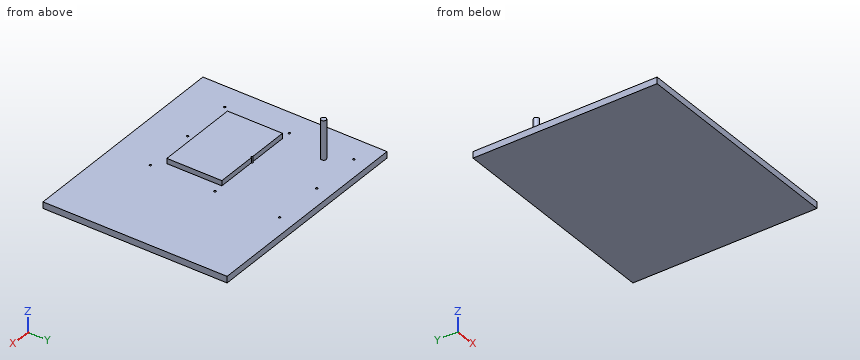
from build123d import *

# Parameters (mm, degrees)
F0_W     = 860
F0_H     = 713
F1_DEPTH = 25
F2_R     = 4
F3_DEPTH = 20
F5_DEPTH = 20
F6_R     = 10
F7_DEPTH = 150


with BuildPart() as f1:
    # F0 (on Top) → F1 (new body)
    with BuildSketch(Plane.XY):
        with Locations((-372.361999, 315.663677)):
            Rectangle(F0_W, F0_H)
    extrude(amount=-F1_DEPTH)

    # F2 (on face) → F3 (cut)
    with BuildSketch(Plane.XY):
        with Locations((-706.361999, 613.163677)):
            Circle(F2_R)
        with Locations((-506.361999, 613.163677)):
            Circle(F2_R)
        with Locations((-306.361999, 613.163677)):
            Circle(F2_R)
        with Locations((-706.361999, 363.163677)):
            Circle(F2_R)
        with Locations((-506.361999, 363.163677)):
            Circle(F2_R)
        with Locations((-306.361999, 363.163677)):
            Circle(F2_R)
        with Locations((-706.361999, 113.163677)):
            Circle(F2_R)
        with Locations((-506.361999, 113.163677)):
            Circle(F2_R)
        with Locations((-306.361999, 113.163677)):
            Circle(F2_R)
    extrude(amount=-F3_DEPTH, mode=Mode.SUBTRACT)

    # F4 (on face) → F5 (join)
    with BuildSketch(Plane.XY):
        with BuildLine():
            Line((-669.361999, 363.163677), (-669.361999, 150.163677))
            Line((-669.361999, 150.163677), (-343.272001, 150.163677))
            Line((-343.272001, 150.163677), (-343.272001, 363.163677))
            Line((-343.272001, 363.163677), (-502.361999, 363.163677))
            ThreePointArc((-502.361999, 363.163677), (-506.361999, 359.163677), (-510.361999, 363.163677))
            Line((-510.361999, 363.163677), (-669.361999, 363.163677))
        make_face()
    extrude(amount=F5_DEPTH)

    # F6 (on face) → F7 (join)
    with BuildSketch(Plane.XY):
        with Locations((-654.361999, 533.163677)):
            Circle(F6_R)
    extrude(amount=F7_DEPTH)


solid = f1.part
Geometry check sheet. Reference: the model listing, model coordinates, mm. Round coordinates to 2 decimals unless told otherwise and drop trailing zeros. Order: outer loops, then holes, each group sorted by start corner. A loop starts at its lowest first (then second) coordinate and runs counter-clockwise, first axis right, second up. Notation, with made-up numbers: M 43,24 L 91,24 A34 ccw 91,61 Z; hole C -32.75,50 d3. An arc over 180 degrees is marked long. Answer in a Markdown table with one row per item.
(1) Go/stop test with flat-tipped pins: P1, Ø13, axis at x = -706.36, y = 113.16, coming from the +Z side; P2, Ø10, axis at x = -413, z = 13, coming from the +Y side; P3, Ø6.5, axis at x = -306.36, y = 613.16, coming from the +Z side; P4, Ø22, axis at y = 213.5, z = 7, coming from the -X side. Record where each tip stops, or that it passes through.
Responses:
| item | result |
|---|---|
| P1 | stops at z = 0 |
| P2 | stops at y = 363.16 |
| P3 | stops at z = -20 |
| P4 | stops at x = -802.36 |
(2) Sectioned sample at A-A, the plane y = 226. Record the cut outline in (x, z).
Responses:
| item | result |
|---|---|
| outline | M -802.36,-25 L 57.64,-25 L 57.64,0 L -343.27,0 L -343.27,20 L -669.36,20 L -669.36,0 L -802.36,0 Z |
(3) Sectioned sample at B-B, the plane x = -402. Record the cut outline in (y, z).
Responses:
| item | result |
|---|---|
| outline | M -40.84,-25 L 672.16,-25 L 672.16,0 L 363.16,0 L 363.16,20 L 150.16,20 L 150.16,0 L -40.84,0 Z |
(4) Sectioned sample at D-D, the plane x = -131.5. Record the cut outline in (y, z).
Responses:
| item | result |
|---|---|
| outline | M -40.84,-25 L 672.16,-25 L 672.16,0 L -40.84,0 Z |
(5) Sectioned sample at C-C, the plane z = 107.5. Record the cut outline in (x, y), and give its area (3 significant figures).
Responses:
| item | result |
|---|---|
| outline | C -654.36,533.16 d20 |
| area | 314 mm² |
(6) Scan lines: probe 1 along Y at (x, z) = (-653.5, 36.5); probe 2 along Z at (x, y) = (-539, 161.5); probe 3 along Z at (x, y) = (-323, 478.5). Record each from-to range of solid material in increasing order. Write a range as from..to.
Responses:
| item | result |
|---|---|
| probe 1 | y = 523.2..543.13 |
| probe 2 | z = -25..20 |
| probe 3 | z = -25..0 |
